```python
from build123d import *

# Parameters (mm, degrees)
SKETCH2_W           = 465.25
SKETCH2_H           = 140
SKETCH2_W_2         = 29.5
BOSS_EXTRUDE3_DEPTH = 5
FILLET1_R           = 4
SKETCH5_W           = 20.1
SKETCH5_H           = 20.1
CUT_EXTRUDE1_DEPTH  = 2.5
CUT_EXTRUDE2_DEPTH  = 10


with BuildPart() as part:
    # Sketch2 → Boss-Extrude3 (new body)
    # profile 1 of 3: a face of its own
    with BuildSketch(Plane.XY.offset(-537.770775127)):
        with Locations((-247.493842126, 630)):
            Rectangle(SKETCH2_W, SKETCH2_H)
        with BuildLine():
            Line((-456.868842126, 675.75), (-456.868842126, 584.25))
            ThreePointArc((-456.868842126, 584.25), (-461.118842126, 580), (-465.368842126, 584.25))
            Line((-465.368842126, 584.25), (-465.368842126, 675.75))
            ThreePointArc((-465.368842126, 675.75), (-461.118842126, 680), (-456.868842126, 675.75))
        make_face(mode=Mode.SUBTRACT)
        with BuildLine():
            ThreePointArc((-416.868842126, 584.25), (-421.118842126, 580), (-425.368842126, 584.25))
            Line((-425.368842126, 584.25), (-425.368842126, 675.75))
            ThreePointArc((-425.368842126, 675.75), (-421.118842126, 680), (-416.868842126, 675.75))
            Line((-416.868842126, 675.75), (-416.868842126, 584.25))
        make_face(mode=Mode.SUBTRACT)
        with BuildLine():
            Line((-15.868842127, 675.75), (-15.868842127, 584.25))
            ThreePointArc((-15.868842127, 584.25), (-20.118842127, 580), (-24.368842127, 584.25))
            Line((-24.368842127, 584.25), (-24.368842127, 675.75))
            ThreePointArc((-24.368842127, 675.75), (-20.118842127, 680), (-15.868842127, 675.75))
        make_face(mode=Mode.SUBTRACT)
    # profile 2 of 3: a face of its own
    with BuildSketch(Plane.XY.offset(-537.770775127)):
        with Locations((-0.118842126, 630)):
            Rectangle(SKETCH2_W_2, SKETCH2_H)
    # profile 3 of 3: a face of its own
    with BuildSketch(Plane.XY.offset(-537.770775127)):
        Polygon((15.631157874, 700), (14.631157874, 700), (14.631157874, 560), (38.881157874, 560), (38.881157874, 700), (24.131157874, 700), align=None)
        with BuildLine():
            ThreePointArc((24.131157874, 584.25), (19.881157874, 580), (15.631157874, 584.25))
            Line((15.631157874, 584.25), (15.631157874, 675.75))
            ThreePointArc((15.631157874, 675.75), (19.881157874, 680), (24.131157874, 675.75))
            Line((24.131157874, 675.75), (24.131157874, 584.25))
        make_face(mode=Mode.SUBTRACT)
    extrude(amount=BOSS_EXTRUDE3_DEPTH)

    # Fillet1
    fillet1_edges = [part.edges().sort_by_distance(p)[0] for p in [
        (-480.118842126, 700, -535.270775127),
        (38.881157874, 700, -535.270775127),
        (38.881157874, 560, -535.270775127),
        (-480.118842126, 560, -535.270775127),
    ]]
    fillet(fillet1_edges, radius=FILLET1_R)

    # Sketch5 → Cut-Extrude1 (cut)
    with BuildSketch(Plane.XY.offset(-532.770775127)):
        with Locations((-220.568842126, 629.95)):
            Rectangle(SKETCH5_W, SKETCH5_H)
    extrude(amount=-CUT_EXTRUDE1_DEPTH, mode=Mode.SUBTRACT)

    # Sketch6 → Cut-Extrude2 (cut)
    with BuildSketch(Plane.XY.offset(-532.770775127)):
        with BuildLine():
            Line((-191.098842126, 632.575), (-202.552234041, 632.575))
            ThreePointArc((-202.552234041, 632.575), (-205.127234041, 630), (-202.552234041, 627.425))
            Line((-202.552234041, 627.425), (-191.098842126, 627.425))
            ThreePointArc((-191.098842126, 627.425), (-188.523842126, 630), (-191.098842126, 632.575))
        make_face()
        with BuildLine():
            Line((-250.138842126, 627.425), (-238.685450212, 627.425))
            ThreePointArc((-238.685450212, 627.425), (-236.110450212, 630), (-238.685450212, 632.575))
            Line((-238.685450212, 632.575), (-250.138842126, 632.575))
            ThreePointArc((-250.138842126, 632.575), (-252.713842126, 630), (-250.138842126, 627.425))
        make_face()
    extrude(amount=-CUT_EXTRUDE2_DEPTH, mode=Mode.SUBTRACT)


solid = part.part
```
The listing builds one solid part. Answer for the finished solid, in the listing's coordinates (mm). Give positions to 0.01 mm unless a question says otherwise; leave off trailing zeros. Loops run counter-clockwise (first coordinate to the right, second up) from the corner with the lowest first, then second, coordinate; pieces in that order, holes last. Notation, with made-up numbers: M -15,12 L 28,12 A13 ccw 28,23 Z; hole C 20.5,-21.75 d3. An arc over 180 degrees is marked long. One line per item, written item: value.
1. For a pull along Y with two mould halves and no side action, classify faces 1 (the face through (-224, 647, -532.771)), 2 (the face through (-221, 630, -535.271)) as pulls with the +Y half, pulls with the -Y half, needs draft (parallel to the pull), parting line crosses it, or undercut.
Found:
face 1: needs draft
face 2: undercut
2. Find the intervals of material crossed by probe 1 along X at (y, z) = (592.5, -536.1); probe 2 along Y at (x, z) = (-236.5, -536.55); probe 3 along Y at (x, z) = (-419, -537.5), in increasing order.
Found:
probe 1: -480.12 to -465.37, -456.87 to -425.37, -416.87 to -24.37, -15.87 to 15.63, 24.13 to 38.88
probe 2: 560 to 628.64, 631.36 to 700
probe 3: 560 to 580.57, 679.43 to 700
3. This flat-tipped pin is pushed along its axis until it touches: P1, Ø6, axis at x = -223.5, y = 628, coming from the +Z side. Where does it stop, or does it pass through?
Found:
P1: z = -535.27
4. Section A-A on y = 614 is taken. Determine the outline of the cut face in (x, z), plus the area to 4 significant figures.
Found:
outline: M -480.12,-537.77 L -465.37,-537.77 L -465.37,-532.77 L -480.12,-532.77 Z; M -456.87,-537.77 L -425.37,-537.77 L -425.37,-532.77 L -456.87,-532.77 Z; M -416.87,-537.77 L -24.37,-537.77 L -24.37,-532.77 L -416.87,-532.77 Z; M -15.87,-537.77 L 15.63,-537.77 L 15.63,-532.77 L -15.87,-532.77 Z; M 24.13,-537.77 L 38.88,-537.77 L 38.88,-532.77 L 24.13,-532.77 Z
area: 2,425 mm^2
5. Section B-B on z = -533.8 is taken. State how many separate pieces and enclosed holes the cut face has, plus the area to 3 significant figures.
Found:
separate pieces: 1
enclosed holes: 7
area: 68,700 mm^2
